```python
from build123d import *

# Parameters (mm, degrees)
CHAMFER_1_SIZE = 0.5


with BuildPart() as part:
    # Эскиз1 → Revolve 325 (revolve)
    with BuildSketch(Plane(origin=(0, 0, 0), x_dir=(1, 0, 0), z_dir=(0, 1, 0)), mode=Mode.PRIVATE) as revolve_325_sk:
        Polygon((0, 0), (8, 0), (8, 5), (3, 5), (3, 6), (2, 6), (2, 9), (0, 9), align=None)
    revolve(revolve_325_sk.sketch.rotate(Axis((0, 0, -9), (0, 0, 1)), 180), axis=Axis((0, 0, -9), (0, 0, 1)))

    # Фаска1
    chamfer_1_edges = [part.edges().sort_by_distance(p)[0] for p in [
        (2, 0, -9),
    ]]
    chamfer(chamfer_1_edges, length=CHAMFER_1_SIZE)


solid = part.part
```
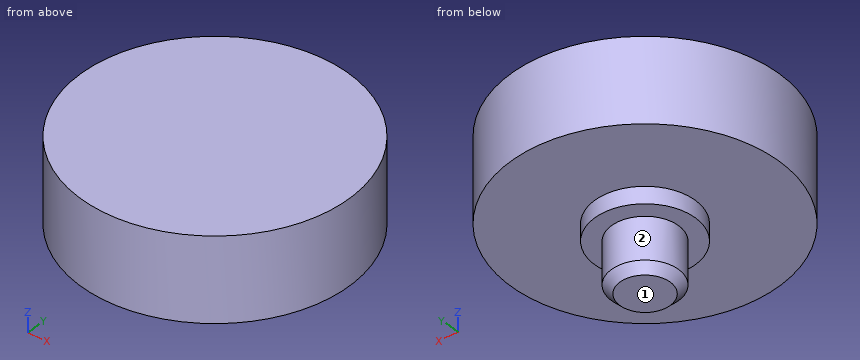
Input: part model. Units: mm. Frame: model coordinates. Face numbers are marked on the shaded views. A direction names the side the tool comes from. Give positions to 0.01 mm unless a question says otherwise; leave off trailing zeros. Order: outer loops, then holes, each group sorted by start corner. A loop starts at its lowest first (then second) coordinate and runs counter-clockwise, first axis right, second up. Notation, with made-up numbers: (2.5, 29) -> (37.5, 29) arc R28 ccw to (37.5, 67) -> close; hole circle Ø11 at (66, -36). An arc over 180 degrees is marked (long way). Write each question's results on one line, items separated by ' | '. Start each with the question number.
Item 1: Cut plane D-D on z = -6.75. Return the cut outline in (x, y), then the cut area to 3 significant figures.
Item 2: Line query: line 1 (Z direction, x = -1, y = -4); line 2 (Y direction, x = 0, z = -7); line 3 (Z direction, x = -0.5, y = 2.25). Output: solid intervals per line, ascending.
Item 3: Cut plane C-C on z = -3. Return the cut outline in (x, y).
Item 4: Contact query for flat-ended pins moving along their axis: P1, Ø3, axis at x = -2.5, z = -1.5, coming from the -Y side; P2, Ø5, axis at x = 5, z = -2.5, coming from the -Y side; P3, Ø3, axis at x = 5.5, y = -4, coming from the -Z side; P4, Ø3, axis at y = -4.5, z = -7.5, coming from the +X side. Output: stop coordinate, or through.
Item 5: Cut plane A-A on y = 0. Return the cut outline in (x, z), then the cut area to 4 significant figures.
Item 6: Set-up query: the marked faces 1 and 2. Return all of +Z, -Z, +X, -X, +Y, -Y with unobstructed straight access to the full face (end or side cutting, diameter ignored); none if empty.
Established:
1) outline: circle Ø4 at (0, 0) | area: 12.6 mm^2
2) line 1: -5 to 0 | line 2: -2 to 2 | line 3: -6 to 0
3) outline: circle Ø16 at (0, 0)
4) P1: y = -7.94 | P2: y = -7.6 | P3: z = -5 | P4: through
5) outline: (-8, -5) -> (-3, -5) -> (-3, -6) -> (-2, -6) -> (-2, -8.5) -> (-1.5, -9) -> (1.5, -9) -> (2, -8.5) -> (2, -6) -> (3, -6) -> (3, -5) -> (8, -5) -> (8, 0) -> (-8, 0) -> close | area: 97.75 mm^2
6) face 1: -Z, +X, -X, +Y, -Y | face 2: -Z
